Autodesk Inventor part; units mm, degrees
ref_plane "YZ Plane" through (0, 0, 0) normal (1, 0, 0) x (0, 1, 0)
ref_plane "XZ Plane" through (0, 0, 0) normal (0, 1, 0) x (-1, 0, 0)
ref_plane "XY Plane" through (0, 0, 0) normal (0, 0, 1) x (1, 0, 0)
sketch "Sketch2" plane through (0, 0, 0) normal (0, 1, 0) x (-1, 0, 0)
  line L0 (-49, 26.5) -> (49, 26.5)
  line L1 (49, 26.5) -> (49, -26.5)
  line L2 (49, -26.5) -> (-49, -26.5)
  line L3 (-49, -26.5) -> (-49, 26.5)
  point P0 (0, 0)
  point P1 (0, -26.5)
  point P2 (49, 0)
  dimension "d5" = 98
  dimension "d7" = 53
extrude "Extrusion1" add sketch "Sketch2" along normal blind 2
sketch "Sketch3" plane through (0, 2, 0) normal (0, 1, 0) x (1, 0, 0)
  line L0 (-49, -26.5) -> (49, -26.5)
  line L1 (49, -26.5) -> (49, 26.5)
  line L2 (49, 26.5) -> (-49, 26.5)
  line L3 (-49, 26.5) -> (-49, -26.5)
  arc A0 (43.75, 17.5) -> (43.75, 23) centre (43.75, 20.25) ccw
  arc A1 (41.25, 23) -> (41.25, 17.5) centre (41.25, 20.25) ccw
  line L4 (41.25, 23) -> (43.75, 23)
  line L5 (41.25, 17.5) -> (43.75, 17.5)
  arc A2 (-41.25, 17.5) -> (-41.25, 23) centre (-41.25, 20.25) ccw
  arc A3 (-43.75, 23) -> (-43.75, 17.5) centre (-43.75, 20.25) ccw
  line L6 (-43.75, 23) -> (-41.25, 23)
  line L7 (-43.75, 17.5) -> (-41.25, 17.5)
  arc A4 (43.75, -23) -> (43.75, -17.5) centre (43.75, -20.25) ccw
  arc A5 (41.25, -17.5) -> (41.25, -23) centre (41.25, -20.25) ccw
  line L8 (41.25, -17.5) -> (43.75, -17.5)
  line L9 (41.25, -23) -> (43.75, -23)
  arc A6 (-41.25, -23) -> (-41.25, -17.5) centre (-41.25, -20.25) ccw
  arc A7 (-43.75, -17.5) -> (-43.75, -23) centre (-43.75, -20.25) ccw
  line L10 (-43.75, -17.5) -> (-41.25, -17.5)
  line L11 (-43.75, -23) -> (-41.25, -23)
  point P0 (0, 0)
  dimension "d10" = 5.5
  dimension "d13" = 2.5
  dimension "d14" = 20.25
  dimension "d15" = 41.25
  dimension "d20" = 85
  dimension "d23" = 40.5
extrude "Extrusion4" cut sketch "Sketch3" against normal blind 2 keep common part
sketch "Sketch4" plane through (0, 2, 0) normal (0, 1, 0) x (1, 0, 0)
  circle A0 centre (0, 0) radius 19
  dimension "d30" = 38
extrude "Extrusion5" add sketch "Sketch4" along normal blind 2
sketch "Sketch5" plane through (0, 4, 0) normal (0, 1, 0) x (1, 0, 0)
  circle A0 centre (0, 0) radius 19
  circle A1 centre (0, 0) radius 4
  dimension "d34" = 8
extrude "Extrusion6" add sketch "Sketch5" along normal blind 46 contours A1
sketch "Sketch6" plane through (0, 0, 0) normal (0, -1, 0) x (1, 0, 0)
  line L0 (-32.5, 31) -> (32.5, 31)
  line L1 (32.5, 31) -> (32.5, -31)
  line L2 (32.5, -31) -> (-32.5, -31)
  line L3 (-32.5, -31) -> (-32.5, 31)
  point P0 (0, 0)
  point P1 (0, 31)
  point P2 (-32.5, 0)
  dimension "d39" = 65
  dimension "d42" = 62
extrude "Extrusion7" add sketch "Sketch6" along normal blind 36
sketch "Sketch7" plane through (0, 50, 0) normal (0, 1, 0) x (1, 0, 0)
  circle A0 centre (0, 0) radius 4
  circle A1 centre (0, 0) radius 18
  line L0 (11.079, 14.1865) -> (-11.079, -14.1865)
  dimension "d46" = 36
revolve "Revolution1" add sketch "Sketch7" angle 360 about axis through (11.079, 50, -14.1865) along (-0.6154984, 0, 0.7881381) picked at (-1.4546, 2.0706) picked at (6.9677, 11.2549) contours L0 A0 | A0 L0 A1
fillet "Fillet1" radius 2 1 edges at (49, 1, 26.5)
fillet "Fillet2" radius 2 1 edges at (49, 1, -26.5)
fillet "Fillet3" radius 2 1 edges at (-49, 1, -26.5)
fillet "Fillet4" radius 2 1 edges at (-49, 1, 26.5)
fillet "Fillet5" radius 2 1 edges at (-19, 4, 0)
equation "\"BendRadius\" = Thickness"
equation "\"BendReliefWidth\" = Thickness"
equation "\"BendReliefDepth\" = 0.5 * Thickness"
equation "\"CornerReliefSize\" = 4 * Thickness"
equation "\"MinimumRemnant\" = 2 * Thickness"
equation "\"TransitionRadius\" = BendRadius"
equation "\"JacobiRadiusSize\" = Thickness"
equation "\"GapSize\" = Thickness"
properties part number "Sanwa_Joystick_JLF-TP-8YT"
Design review of the part built by this model. Coordinates are the model's own, in mm. A direction names the side the tool comes from. Round coordinates to 2 decimals unless told otherwise and drop trailing zeros. Write each loop counter-clockwise with the first axis right and the second up, starting at its lowest first coordinate (ties: lowest second). Pieces come first, ordered by that corner, then holes. Notation, with made-up numbers: M 31,59 L 56,59 A10 cw 56,67 Z; hole C -0.75,11.25 d3. An arc over 180 degrees is marked long. One line per item, written item: value. Start each with the question number.
1. Draft analysis for pull direction X (two halves, no side actions). For faces 1 (the face through (0, -36, 0)), 2 (the face through (32.5, -18, 0)), 3 (the face through (-38.5, 1, 20.3)), state which applies: pulls with the +X half, pulls with the -X half, needs draft (parallel to the pull), parting line crosses it, or undercut.
2. For faces 4 (the face through (38.5, 1, 20.2)), 5 (the face through (41, 0, 0)), 6 (the face through (-0.867, 18.026, -3.905)), 7 (the face through (0, 0, 29)), list the 3-axis set-ups (+Z, -Z, +X, -X, +Y, -Y) from which the entire face can be reached by the end or side of a thin tool; tool diameter is ignored.
3. Clearance check with flat-ended pins moving along their axes: P1, Ø1.5, axis at y = 30.5, z = -1.5, coming from the +X side; P2, Ø2, axis at x = -42.5, y = 1, coming from the -Z side; P3, Ø2, axis at x = -42.5, y = 1, coming from the +Z side. State where each tip first meets the part, or that it passes through.
4. Take a section at C-C on z = 21. State the section outline as (x, y) points, then the cut area to 3 significant figures.
5. Take a section at A-A on z = -20.25. State the section outline as (x, y) points, then the cut area to 3 significant figures.
6. To check wall thickness, follow probe 1 along Y at (x, z) = (-20, 11.5); probe 2 along Y at (x, z) = (-41, 15); probe 3 along X at (y, z) = (-3, 24). State the ranges of each line that lie inside material, in increasing order. Write a range as from..to.
7. Take a section at D-D on y = 19.5. State the section outline as (x, z) points, then the cut area to 3 significant figures.
Computed:
1. face 1: needs draft
1. face 2: pulls with the +X half
1. face 3: undercut
2. face 4: +Y, -Y
2. face 5: +Z, -Z, +X, -Y
2. face 6: none
2. face 7: +Z, +X, -X, +Y
3. P1: stops at x = 3.93
3. P2: stops at z = -26.5
3. P3: stops at z = 26.5
4. outline: M -49,0 L -46.4,0 L -46.4,2 L -49,2 Z; M -38.6,0 L -32.5,0 L -32.5,-36 L 32.5,-36 L 32.5,0 L 38.6,0 L 38.6,2 L -38.6,2 Z; M 46.4,0 L 49,0 L 49,2 L 46.4,2 Z
4. area: 2,500 mm²
5. outline: M -49,0 L -46.5,0 L -46.5,2 L -49,2 Z; M -38.5,0 L -32.5,0 L -32.5,-36 L 32.5,-36 L 32.5,0 L 38.5,0 L 38.5,2 L -38.5,2 Z; M 46.5,0 L 49,0 L 49,2 L 46.5,2 Z
5. area: 2,500 mm²
6. probe 1: y = -36..2
6. probe 2: y = 0..2
6. probe 3: x = -32.5..32.5
7. outline: C 0,0 d8
7. area: 50.3 mm²
